Autodesk Inventor part; units mm, degrees
ref_plane "YZ Plane" through (0, 0, 0) normal (1, 0, 0) x (0, 1, 0)
ref_plane "XZ Plane" through (0, 0, 0) normal (0, 1, 0) x (-1, 0, 0)
ref_plane "XY Plane" through (0, 0, 0) normal (0, 0, 1) x (1, 0, 0)
sketch "스케치3" plane through (0, 0, 0) normal (0, 1, 0) x (-1, 0, 0)
  line L0 (35.7919, -14.8255) -> (14.8255, -35.7919)
  line L1 (14.8255, -35.7919) -> (-14.8255, -35.7919)
  line L2 (-14.8255, -35.7919) -> (-35.7919, -14.8255)
  line L3 (-35.7919, -14.8255) -> (-35.7919, 14.8255)
  line L4 (-35.7919, 14.8255) -> (-14.8255, 35.7919)
  line L5 (-14.8255, 35.7919) -> (14.8255, 35.7919)
  line L6 (14.8255, 35.7919) -> (35.7919, 14.8255)
  line L7 (35.7919, 14.8255) -> (35.7919, -14.8255)
  line L8 (13.5, -32.5919) -> (-13.5, -32.5919)
  line L9 (-13.5, -32.5919) -> (-32.5919, -13.5)
  line L10 (-32.5919, -13.5) -> (-32.5919, 13.5)
  line L11 (-32.5919, 13.5) -> (-13.5, 32.5919)
  line L12 (-13.5, 32.5919) -> (13.5, 32.5919)
  line L13 (13.5, 32.5919) -> (32.5919, 13.5)
  line L14 (32.5919, 13.5) -> (32.5919, -13.5)
  line L15 (32.5919, -13.5) -> (13.5, -32.5919)
  point P0 (0, 0)
  point P1 (0, 0)
  point P2 (0, 0)
  point P3 (0, 0)
  dimension "d66" = 27
  dimension "d67" = 3.2
extrude "돌출2" add sketch "스케치3" along normal blind 4.4 contours L0 L1 L2 L3 L4 L5 L6 L7 | L8 L9 L10 L11 L12 L13 L14 L15
sketch "스케치4" plane through (0, 4.4, 0) normal (0, 1, 0) x (1, 0, 0)
  line L0 (13.5, -32.5919) -> (-13.5, -32.5919)
  line L1 (-13.5, -32.5919) -> (-32.5919, -13.5)
  line L2 (-32.5919, -13.5) -> (-32.5919, 13.5)
  line L3 (-32.5919, 13.5) -> (-13.5, 32.5919)
  line L4 (-13.5, 32.5919) -> (13.5, 32.5919)
  line L5 (13.5, 32.5919) -> (32.5919, 13.5)
  line L6 (32.5919, 13.5) -> (32.5919, -13.5)
  line L7 (32.5919, -13.5) -> (13.5, -32.5919)
  line L8 (-14.1627, 34.1919) -> (14.1627, 34.1919)
  line L9 (14.1627, 34.1919) -> (34.1919, 14.1627)
  line L10 (34.1919, 14.1627) -> (34.1919, -14.1627)
  line L11 (34.1919, -14.1627) -> (14.1627, -34.1919)
  line L12 (14.1627, -34.1919) -> (-14.1627, -34.1919)
  line L13 (-14.1627, -34.1919) -> (-34.1919, -14.1627)
  line L14 (-34.1919, -14.1627) -> (-34.1919, 14.1627)
  line L15 (-34.1919, 14.1627) -> (-14.1627, 34.1919)
  line L16 (-13.3343, 32.1919) -> (13.3343, 32.1919)
  line L17 (13.3343, 32.1919) -> (32.1919, 13.3343)
  line L18 (32.1919, 13.3343) -> (32.1919, -13.3343)
  line L19 (32.1919, -13.3343) -> (13.3343, -32.1919)
  line L20 (13.3343, -32.1919) -> (-13.3343, -32.1919)
  line L21 (-13.3343, -32.1919) -> (-32.1919, -13.3343)
  line L22 (-32.1919, -13.3343) -> (-32.1919, 13.3343)
  line L23 (-32.1919, 13.3343) -> (-13.3343, 32.1919)
  line L24 (-14.8255, 35.7919) -> (-35.7919, 14.8255)
  point P0 (0, 0)
  point P1 (0, 0)
  point P2 (0, 0)
  point P3 (0, 0)
  dimension "d7" = 27
  dimension "d99" = 1.6
  dimension "d100" = 2
extrude "돌출3" cut sketch "스케치4" against normal blind 1.2 contours L0 L1 L2 L3 L4 L5 L6 L7 | L8 L9 L10 L11 L12 L13 L14 L15 | L16 L17 L18 L19 L20 L21 L22 L23
sketch "스케치9" plane through (0, 0, 0) normal (0, -1, 0) x (1, 0, 0)
  line L0 (7.5, 10) -> (2.5, 10)
  line L1 (2.5, 10) -> (2.5, -10)
  line L2 (2.5, -10) -> (7.5, -10)
  line L3 (7.5, -10) -> (7.5, 10)
  line L4 (7.5, 10) -> (2.5, -10) construction
  line L5 (2.5, 10) -> (7.5, -10) construction
  line L6 (-2.5, 10) -> (-7.5, 10)
  line L7 (-7.5, 10) -> (-7.5, -10)
  line L8 (-7.5, -10) -> (-2.5, -10)
  line L9 (-2.5, 10) -> (-7.5, -10) construction
  line L10 (-7.5, 10) -> (-2.5, -10) construction
  line L11 (-2.5, -10) -> (-2.5, 10)
  point P0 (0, 0)
  point P1 (5, 0)
  point P2 (-5, 0)
  dimension "d42" = 20
  dimension "d43" = 5
  dimension "d44" = 2.5
  dimension "d47" = 10
extrude "돌출8" add sketch "스케치9" along normal blind 10
sketch "스케치10" plane through (-7.5, 0, -10) normal (-1, 0, 0) x (0, 0, 1)
  circle A0 centre (15, -5) radius 1.25
  line L0 (19.9591, 0) -> (0.0886, 0)
  line L1 (24.8255, 0) -> (-4.8255, 0)
  circle A1 centre (5, -5) radius 1.25
  line L2 (20, 0) -> (20, -10)
  point P0 (10, 0)
  dimension "d54" = 2.5
  dimension "d57" = 10
  dimension "d62" = 5
  dimension "d63" = 5
extrude "돌출9" cut sketch "스케치10" against normal blind 20
sketch "스케치11" plane through (0, 3.2, 0) normal (0, 1, 0) x (1, 0, 0)
  line L0 (-13.3343, 32.1919) -> (13.3343, 32.1919)
  line L1 (13.3343, 32.1919) -> (32.1919, 13.3343)
  line L2 (32.1919, 13.3343) -> (32.1919, -13.3343)
  line L3 (32.1919, -13.3343) -> (13.3343, -32.1919)
  line L4 (13.3343, -32.1919) -> (-13.3343, -32.1919)
  line L5 (-13.3343, -32.1919) -> (-32.1919, -13.3343)
  line L6 (-32.1919, -13.3343) -> (-32.1919, 13.3343)
  line L7 (-32.1919, 13.3343) -> (-13.3343, 32.1919)
  line L8 (-14.1627, 34.1919) -> (14.1627, 34.1919)
  line L9 (-12.0917, 29.1919) -> (12.0917, 29.1919)
  line L10 (12.0917, 29.1919) -> (29.1919, 12.0917)
  line L11 (29.1919, 12.0917) -> (29.1919, -12.0917)
  line L12 (29.1919, -12.0917) -> (12.0917, -29.1919)
  line L13 (12.0917, -29.1919) -> (-12.0917, -29.1919)
  line L14 (-12.0917, -29.1919) -> (-29.1919, -12.0917)
  line L15 (-29.1919, -12.0917) -> (-29.1919, 12.0917)
  line L16 (-29.1919, 12.0917) -> (-12.0917, 29.1919)
  point P0 (0, 0)
  point P1 (0, 0)
  point P2 (0, 0)
  dimension "d70" = 2
  dimension "d71" = 3
extrude "돌출10" add sketch "스케치11" along normal blind 0.6 contours L0 L1 L2 L3 L4 L5 L6 L7 | L9 L10 L11 L12 L13 L14 L15 L16
fillet "모깎기1" radius 1.2 16 edges at (-25.3087, 4.4, 25.3087) (0, 4.4, 35.7919) (25.3087, 4.4, 25.3087) (35.7919, 4.4, 0) (25.3087, 4.4, -25.3087) (0, 4.4, -35.7919) (-25.3087, 4.4, -25.3087) (-35.7919, 4.4, 0) (-25.3087, 0, 25.3087) (0, 0, 35.7919) (25.3087, 0, 25.3087) (35.7919, 0, 0) (25.3087, 0, -25.3087) (0, 0, -35.7919) (-25.3087, 0, -25.3087) (-35.7919, 0, 0)
properties part number "OV-PAM_bottom_2"
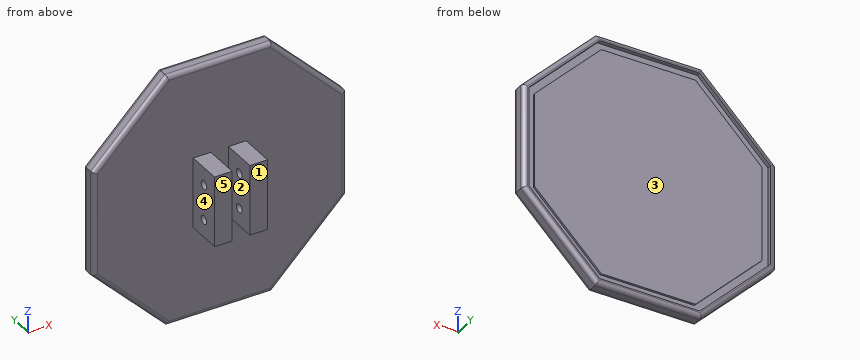
Can you work these out from the model? Positions are in its coordinate system, mm. Face numbers are marked on the shaded views. A direction names the side the tool comes from. Give positions to 0.01 mm unless a question says otherwise; leave off trailing zeros. Order: outer loops, then holes, each group sorted by start corner. A loop starts at its lowest first (then second) coordinate and runs counter-clockwise, first axis right, second up. Notation, with made-up numbers: M -31,-10 L 1,-10 A26 ccw 1,12 Z; hole C 46,-24.75 d2. An arc over 180 degrees is marked long. Use one line per item in the form item = value. Start each with the question number.
Item 1: If we section it at A-A (y = -5): Write out the boundary of the cut face in (x, z), then the cut area to 3 significant figures.
Item 2: We'd pull the mould along X, two halves only. Please class the marked faces 3, 4 and 5: +X half, -X half, draft (parallel to the pull), parting line (faces both ways), or undercut.
Item 3: If we section it at B-B (z = 5): State how many separate pieces and enclosed holes the cut face has, then the cut area to 3 significant figures.
Item 4: Will these pins go through, and if not, where does the flat tip stop? pin 1 Ø2 at (y, z) = (-5, 5) entering from +X; pin 2 Ø19.5 at (x, z) = (-5, 13.5) entering from +Y; pin 3 Ø5.5 at (x, y) = (-6, -6) entering from -Z; pin 4 Ø1.5 at (x, y) = (1.5, -0.5) entering from -Z.
Item 5: For the marked faces 1 and 2, which set-ups out of +Z, -Z, +X, -X, +Y, -Y let a thin tool reach every point of the face, with its end or its side?
Item 6: If I drill on line 1 along X through (y, z) = (-8, 5); line 2 along Y through (x, z) = (-4, -5); line 3 along X through (y, z) = (3.5, 8), over which ranges is the centre line in solid material (lowest first)?
Outcome:
q1.outline = M -7.5,-10 L -2.5,-10 L -2.5,-6.25 L -7.5,-6.25 Z; M -7.5,-3.75 L -2.5,-3.75 L -2.5,3.75 L -7.5,3.75 Z; M -7.5,6.25 L -2.5,6.25 L -2.5,10 L -7.5,10 Z; M 2.5,-10 L 7.5,-10 L 7.5,-6.25 L 2.5,-6.25 Z; M 2.5,-3.75 L 7.5,-3.75 L 7.5,3.75 L 2.5,3.75 Z; M 2.5,6.25 L 7.5,6.25 L 7.5,10 L 2.5,10 Z
q1.area = 150 mm2
q2.face_3 = undercut
q2.face_4 = -X half
q2.face_5 = draft
q3.separate_pieces = 3
q3.enclosed_holes = 0
q3.area = 345 mm2
q4.pin_1 = through
q4.pin_2 = 3.8
q4.pin_3 = -10
q4.pin_4 = -35.33
q5.face_1 = +Z, -Z, +X, -X, -Y
q5.face_2 = +Z, -Z, -Y
q6.line_1 = -7.5 to -2.5, 2.5 to 7.5
q6.line_2 = -10 to -6.25, -3.75 to 3.8
q6.line_3 = -35.75 to -34.19, -32.19 to 32.19, 34.19 to 35.75
